Check sheet for the modelled part. Datum: model origin and axes. Units: mm. A direction names the side the tool comes from. Give positions to 0.01 mm unless a question says otherwise; leave off trailing zeros. Order: outer loops, then holes, each group sorted by start corner. A loop starts at its lowest first (then second) coordinate and runs counter-clockwise, first axis right, second up.
Item 1: Sectioned sample at C-C on z = -137.5. Record the boundary of the cut face in (x, y).
Item 2: Access from +Z, -Z, +X, -X, +Y, -Y to the whole of each face (thin tool, end or side, straight path). Record for faces 4 (the flat face through (44, 16.154, -85)), 5 (the flat face through (44, 14, -79.121)), 6 (the flat face through (44, 21, -142.875)).
Item 3: Release check for a two-part mould opening along Y. For faces 1 (the flat face through (44, 23.139, -84)), 2 (the cylindrical face through (25.216, 14.007, -80.267)), 3 (the flat face through (44, 18.059, -85)) record: released by +Y, released by -Y, zero draft, split by the parting line, or undercut.
Item 4: Sectioned sample at A-A on y = 17. Record the boundary of the cut face in (x, z).
Item 5: Sectioned sample at B-B on x = 36. Record the boundary of the cut face in (y, z) (3 decimals).
Item 6: Sectioned sample at D-D on y = 10.25. Record the boundary of the cut face in (x, z), and give its area (3 significant figures).
Item 7: Gauge pin test, flat ends, axial feed: P1, Ø1.4, axis at x = 44.45, z = -89.09, coming from the +Y side; P2, Ø6, axis at x = 28, y = 15.5, coming from the +Z side; P3, Ø5, axis at x = 29, y = 19.5, coming from the -Z side; P4, Ø2, axis at y = 13.5, z = -140, coming from the -X side. Record the tip position at first contact, or that the pin passes through.
Item 8: Material ranges on line 1 along Z through (x, y) = (44.45, 8.25); line 2 along Z through (x, y) = (29.5, 11.25) (3 decimals); line 3 along Z through (x, y) = (44.45, 6.75), recorded low to high.
from build123d import *

# Parameters (mm, degrees)
SKETCH2_W               = 88.9
SKETCH2_H               = 152.4
BOSS_EXTRUDE1_DEPTH     = 5.9944
CUT_EXTRUDE2_DEPTH      = 177.535840076
CUT_EXTRUDE2_DEPTH_BACK = 177.535840076
SKETCH4_R               = 2.7305
BOSS_EXTRUDE2_DEPTH     = 101.6
FILLET1_R               = 3.81
FILLET2_R               = 2.54
BOSS_EXTRUDE3_DEPTH     = 20.32
FILLET3_R               = 3.81
FILLET6_R               = 3.81
FILLET7_R               = 2.54
CUT_EXTRUDE3_DEPTH      = 204.596488182
CUT_EXTRUDE3_DEPTH_BACK = 204.596488182
SKETCH7_W               = 2.54
SKETCH7_H               = 152.4
SKETCH8_W               = 86.36
SKETCH8_H               = 152.4
CUT_EXTRUDE4_DEPTH      = 5.9944
SKETCH9_R               = 0.79375
CUT_EXTRUDE5_DEPTH      = 3.175


with BuildPart() as part:
    # Sketch2 → Boss-Extrude1 (new body)
    with BuildSketch(Plane(origin=(0, 0, 0), x_dir=(1, 0, 0), z_dir=(0, 1, 0))):
        with Locations((44.45, 76.2)):
            Rectangle(SKETCH2_W, SKETCH2_H)
    extrude(amount=BOSS_EXTRUDE1_DEPTH)

    # Sketch4 → Cut-Extrude2 (cut, two sides: drawn at the far end of the back side and taken through both)
    with BuildSketch(Plane(origin=(0, 5.9944, 0), x_dir=(1, 0, 0), z_dir=(0, 1, 0)).offset(-CUT_EXTRUDE2_DEPTH_BACK)):
        with Locations(Location((45.72, 109.871331367, 0), (0, 0, 270))):
            Circle(SKETCH4_R)
        with Locations(Location((45.72, 33.671331367, 0), (0, 0, 270))):
            Circle(SKETCH4_R)
    extrude(amount=CUT_EXTRUDE2_DEPTH + CUT_EXTRUDE2_DEPTH_BACK, mode=Mode.SUBTRACT)

    # Sketch5 → Boss-Extrude2 (add)
    with BuildSketch(Plane(origin=(0, 5.9944, 0), x_dir=(1, 0, 0), z_dir=(0, 1, 0))):
        Polygon((18.542, 15.748), (12.446, 15.748), (12.446, 2.54), (76.454, 2.54), (76.454, 15.748), (70.358, 15.748), (70.358, 13.208), (71.374, 13.208), (71.374, 11.43), (70.358, 11.43), (70.358, 7.62), (18.542, 7.62), (18.542, 11.43), (17.526, 11.43), (17.526, 13.208), (18.542, 13.208), align=None)
    extrude(amount=BOSS_EXTRUDE2_DEPTH)

    # Fillet1
    fillet1_edges = [part.edges().sort_by_distance(p)[0] for p in [
        (12.446, 56.7944, -15.748),
        (12.446, 56.7944, -2.54),
        (76.454, 56.7944, -2.54),
        (76.454, 56.7944, -15.748),
    ]]
    fillet(fillet1_edges, radius=FILLET1_R)

    # Fillet2
    fillet2_edges = [part.edges().sort_by_distance(p)[0] for p in [
        (71.501, 5.9944, -15.748),
        (44.45, 5.9944, -2.54),
        (12.446, 5.9944, -9.144),
        (17.399, 5.9944, -15.748),
        (76.454, 5.9944, -9.144),
        (13.561923164, 5.9944, -3.655923164),
        (13.561923164, 5.9944, -14.632076836),
        (75.338076836, 5.9944, -3.655923164),
        (75.338076836, 5.9944, -14.632076836),
    ]]
    fillet(fillet2_edges, radius=FILLET2_R - 0.0001)  # a hair under: the kernel refuses the full size

    # Sketch6 → Boss-Extrude3 (add, symmetric)
    with BuildSketch(Plane.ZY.offset(-44.45)):
        Polygon((-149.86, 5.9944), (-79.121, 5.9944), (-79.121, 23.1394), (-86.106, 23.1394), (-86.106, 18.0594), (-84.201, 18.0594), (-84.201, 16.1544), (-86.106, 16.1544), (-86.106, 11.0744), (-142.875, 11.0744), (-142.875, 16.1544), (-144.78, 16.1544), (-144.78, 18.0594), (-142.875, 18.0594), (-142.875, 23.1394), (-149.86, 23.1394), align=None)
    extrude(amount=BOSS_EXTRUDE3_DEPTH, both=True)

    # Fillet3
    fillet3_edges = [part.edges().sort_by_distance(p)[0] for p in [
        (44.45, 23.1394, -149.86),
        (44.45, 23.1394, -79.121),
    ]]
    fillet(fillet3_edges, radius=FILLET3_R)

    # Fillet6
    fillet6_edges = [part.edges().sort_by_distance(p)[0] for p in [
        (24.13, 12.6619, -149.86),
        (64.77, 12.6619, -79.121),
        (24.13, 23.1394, -84.5185),
        (24.13, 12.6619, -79.121),
        (64.77, 23.1394, -84.5185),
        (64.77, 12.6619, -149.86),
        (64.77, 23.1394, -144.4625),
        (64.77, 22.023476836, -148.744076836),
        (64.77, 22.023476836, -80.236923164),
        (24.13, 23.1394, -144.4625),
        (24.13, 22.023476836, -148.744076836),
        (24.13, 22.023476836, -80.236923164),
    ]]
    fillet(fillet6_edges, radius=FILLET6_R)

    # Fillet7
    fillet7_edges = [part.edges().sort_by_distance(p)[0] for p in [
        (24.13, 5.9944, -114.4905),
        (64.77, 5.9944, -114.4905),
        (44.45, 5.9944, -79.121),
        (44.45, 5.9944, -149.86),
        (25.245923164, 5.9944, -80.236923164),
        (63.654076836, 5.9944, -80.236923164),
        (63.654076836, 5.9944, -148.744076836),
        (25.245923164, 5.9944, -148.744076836),
    ]]
    fillet(fillet7_edges, radius=FILLET7_R - 0.0001)  # a hair under: the kernel refuses the full size

    # Sketch7 → Cut-Extrude3 (cut, two sides: drawn at the far end of the back side and taken through both)
    with BuildSketch(Plane(origin=(0, 5.9944, 0), x_dir=(1, 0, 0), z_dir=(0, 1, 0)).offset(-CUT_EXTRUDE3_DEPTH_BACK)):
        with Locations((1.27, 76.2)):
            Rectangle(SKETCH7_W, SKETCH7_H)
    extrude(amount=CUT_EXTRUDE3_DEPTH + CUT_EXTRUDE3_DEPTH_BACK, mode=Mode.SUBTRACT)

    # Sketch8 → Cut-Extrude4 (cut)
    with BuildSketch(Plane.XZ):
        with Locations((45.72, -76.2)):
            Rectangle(SKETCH8_W, SKETCH8_H)
    extrude(amount=-CUT_EXTRUDE4_DEPTH, mode=Mode.SUBTRACT)


with BuildPart() as body_2:
    # of the pieces the cut leaves, the one that is kept (cut_extrude4_keep)
    add(part.part.solids().sort_by_distance((27.94, 8.5343, -149.86))[0])

    # Sketch9 → Cut-Extrude5 (cut)
    with BuildSketch(Plane.XZ.offset(-5.9944)):
        with Locations(Location((44.45, -89.0905, 0), (0, 0, 270))):
            Circle(SKETCH9_R)
        with Locations(Location((44.45, -139.8905, 0), (0, 0, 270))):
            Circle(SKETCH9_R)
    extrude(amount=-CUT_EXTRUDE5_DEPTH, mode=Mode.SUBTRACT)


solid = body_2.part
Report:
1. outline: (21.59, 5.99) - (67.31, 5.99) arc R2.54 cw to (64.77, 8.53) - (64.77, 11.07) - (24.13, 11.07) - (24.13, 8.53) arc R2.54 cw to start
2. face 4: +X, -X
2. face 5: +Z, +X, -X, +Y
2. face 6: +X, -X, +Y
3. face 1: released by +Y
3. face 2: zero draft
3. face 3: undercut
4. outline: (24.13, -146.05) arc R3.81 ccw to (27.94, -149.86) - (60.96, -149.86) arc R3.81 ccw to (64.77, -146.05) - (64.77, -144.78) - (24.13, -144.78) - close; (24.13, -84.2) - (64.77, -84.2) - (64.77, -82.93) arc R3.81 ccw to (60.96, -79.12) - (27.94, -79.12) arc R3.81 ccw to (24.13, -82.93) - close
5. outline: (5.994, -152.4) arc R2.54 cw to (8.534, -149.86) - (19.329, -149.86) arc R3.81 ccw to (23.139, -146.05) - (23.139, -142.875) - (18.059, -142.875) - (18.059, -144.78) - (16.154, -144.78) - (16.154, -142.875) - (11.074, -142.875) - (11.074, -86.106) - (16.154, -86.106) - (16.154, -84.201) - (18.059, -84.201) - (18.059, -86.106) - (23.139, -86.106) - (23.139, -82.931) arc R3.81 ccw to (19.329, -79.121) - (8.534, -79.121) arc R2.54 cw to (5.994, -76.581) - close
6. outline: (24.13, -146.05) arc R3.81 ccw to (27.94, -149.86) - (60.96, -149.86) arc R3.81 ccw to (64.77, -146.05) - (64.77, -82.93) arc R3.81 ccw to (60.96, -79.12) - (27.94, -79.12) arc R3.81 ccw to (24.13, -82.93) - close
6. area: 2,860 mm2
7. P1: stops at y = 11.07
7. P2: stops at z = -79.12
7. P3: stops at z = -149.86
7. P4: passes through
8. line 1: z = -149.88 to -140.68, -139.1 to -89.88, -88.3 to -79.11
8. line 2: z = -149.86 to -142.875, -86.106 to -79.121
8. line 3: z = -150.59 to -140.68, -139.1 to -89.88, -88.3 to -78.39
